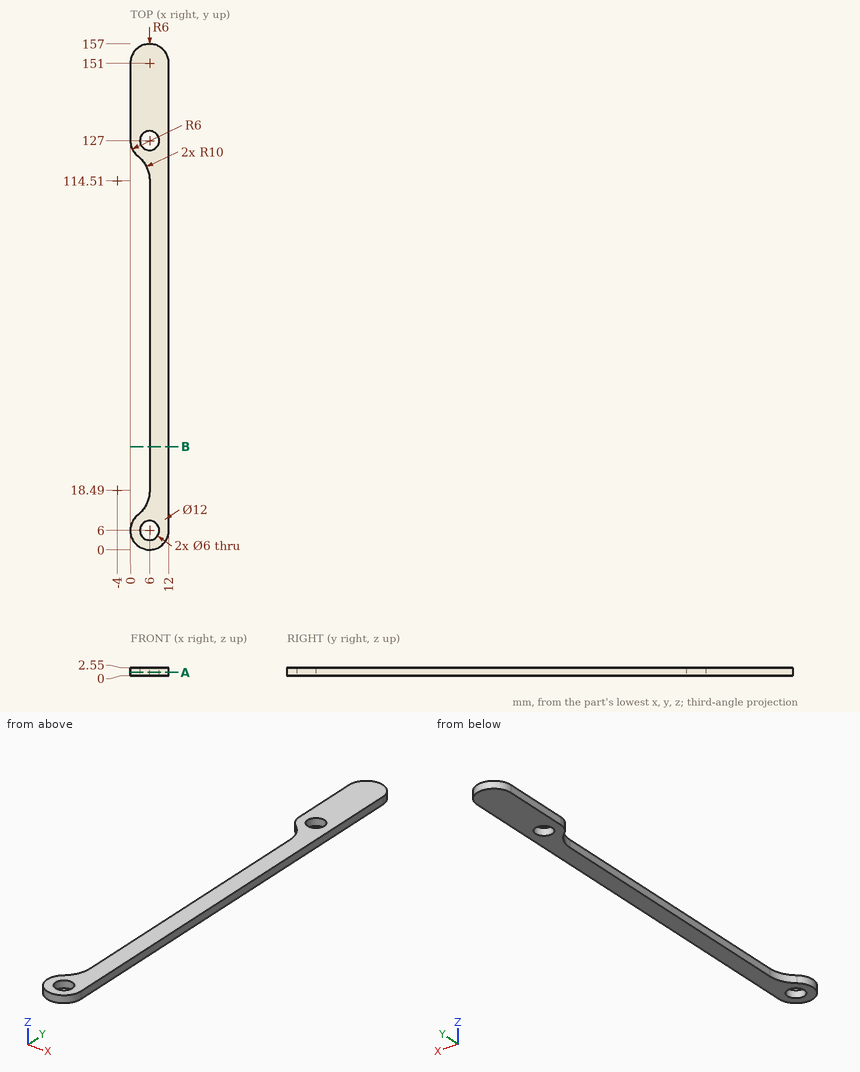
Input: dimensioned drawing with shaded views. Units: mm. Origin: part minimum x, y, z. Coordinates: 2 decimals unless noted, no trailing zeros. Write each loop counter-clockwise with the first axis right and the second up, starting at its lowest first coordinate (ties: lowest second). Pieces come first, ordered by that corner, then holes. Notation, with made-up numbers: M -33.5,21.25 L 12.5,21.25 A28 ccw 12.5,48.25 Z; hole C -9,56 d10. An arc over 180 degrees is marked long. Use one line per item in the form item = value.
Q1. First-contact query: pin 1 (1.3 mm diameter, centred on y = 76.5, z = 0.5, fed in from -X). Flat tip, straight axial feed; report the tip coordinate or a pass-through.
Answer below:
pin_1 = 6
Q2. Section B-B (y = 32). Return loops of the section in (x, z).
Answer below:
outline = M 6,0 L 12,0 L 12,2.55 L 6,2.55 Z
Q3. Material intervals for probe 1 along X at (y, z) = (127, 1.85); probe 2 along Y at (x, z) = (8.5, 2); probe 3 along Y at (x, z) = (4.5, 0.1), sorted ascending. Write a range as from..to.
Answer below:
probe_1 = 0..3, 9..12
probe_2 = 0.55..4.34, 7.66..125.34, 128.66..156.45
probe_3 = 0.19..3.4, 8.6..13.22, 119.78..124.4, 129.6..156.81
Q4. Section A-A (z = 1.1). Return loops of the section in (x, y).
Answer below:
outline = M 0,127 A6 ccw 2.25,122.32 A10 cw 6,114.51 L 6,18.49 A10 cw 2.25,10.68 A6 ccw long 12,6 L 12,151 A6 ccw 0,151 Z; hole C 6,6 d6; hole C 6,127 d6
